```python
from build123d import *

# Parameters (mm, degrees)
SKETCH_1_W         = 20
SKETCH_1_H         = 20
BASEBOX_DEPTH      = 10
SKETCH_2_W         = 10
SKETCH_2_H         = 10
DRAFTOUTWARD_DEPTH = 10
DRAFTOUTWARD_TAPER = 5


with BuildPart() as part:
    # 草图1 → BaseBox (new body)
    with BuildSketch(Plane.XY):
        with Locations((10, 10)):
            Rectangle(SKETCH_1_W, SKETCH_1_H)
    extrude(amount=BASEBOX_DEPTH)

    # 草图2 → DraftOutward (add)
    with BuildSketch(Plane.XY.offset(10)):
        with Locations((10, 10)):
            Rectangle(SKETCH_2_W, SKETCH_2_H)
    extrude(amount=DRAFTOUTWARD_DEPTH, taper=DRAFTOUTWARD_TAPER)


solid = part.part
```
Input: part model. Units: mm. Frame: model coordinates. A direction names the side the tool comes from. Coordinates: 2 decimals unless noted, no trailing zeros. Order: outer loops, then holes, each group sorted by start corner. A loop starts at its lowest first (then second) coordinate and runs counter-clockwise, first axis right, second up. Notation, with made-up numbers: (-34.75, -31.75) - (5.25, -31.75) arc R22 ccw to (5.25, -25.75) - close; hole circle Ø3 at (-26.75, 48.5). An arc over 180 degrees is marked (long way). Return JSON: item names as keys, results as strings.
Q1. Cut plane D-D (y = 18.5). Return loops of the section in (x, z), then the cut area to 3 significant figures.
The answers:
{"outline": "(0, 0) - (20, 0) - (20, 10) - (0, 10) - close", "area": "200 mm2"}
Q2. Cut plane A-A (y = 11.75). Return loops of the section in (x, z).
The answers:
{"outline": "(0, 0) - (20, 0) - (20, 10) - (15, 10) - (14.13, 20) - (5.87, 20) - (5, 10) - (0, 10) - close"}
Q3. Ray query, probe 1 along Z at (x, y) = (11.5, 17.75); probe 2 along X at (y, z) = (10, 15.75); probe 3 along Y at (x, z) = (13.5, 13.5). Return the intervals inside material, ascending.
The answers:
{"probe 1": "z = 0 to 10", "probe 2": "x = 5.5 to 14.5", "probe 3": "y = 5.31 to 14.69"}
Q4. Access query for faces 1 (the flat face through (10, 10, 0)), 2 (the flat face through (3, 10, 10)). Directions: +Z, -Z, +X, -X, +Y, -Y. A direction counts if a zero-diameter tool reaches every point of the face in a straight line with its end or side. Return the directions, or none.
The answers:
{"face 1": "-Z, +X, -X, +Y, -Y", "face 2": "+Z"}
Q5. Cut plane C-C (z = 18.5). Return loops of the section in (x, y).
The answers:
{"outline": "(5.74, 5.74) - (14.26, 5.74) - (14.26, 14.26) - (5.74, 14.26) - close"}
Q6. First-contact query: pin 1 (2 mm diameter, centred on y = 16, z = 14.5, fed in from -X); pin 2 (6 mm diameter, centred on y = 11.5, z = 17, fed in from -X); pin 3 (6 mm diameter, centred on y = 16.5, z = 17.5, fed in from +X). Flat tips, straight axial feed; report the tip coordinate or a pass-through.
The answers:
{"pin 1": "passes through", "pin 2": "stops at x = 5.35", "pin 3": "stops at x = 14.54"}
